For this review, take the finished solid that the model builds, in its own axes (mm). Face numbers are marked on the shaded views. A direction names the side the tool comes from. Round coordinates to 2 decimals unless told otherwise and drop trailing zeros. Write each loop counter-clockwise with the first axis right and the second up, starting at its lowest first coordinate (ties: lowest second). Pieces come first, ordered by that corner, then holes. Notation, with made-up numbers: (62.5, -29.5) -> (95.5, -29.5) arc R9 cw to (95.5, -18.5) -> close; hole circle Ø4 at (-13.5, 29.5). An arc over 180 degrees is marked (long way). Answer as CSV lines item,"result". Start each with the question number.
Item 1: Take a section at A-A on x = 22. Give the boundary of the cut face in (y, z), then the cut area to 3 significant figures.
Item 2: Take a section at B-B on y = 40. Give the boundary of the cut face in (x, z).
Item 3: Machinability: for the marked faces 1, 2, 3, 4 and 5, which of the approach directions +Z, -Z, +X, -X, +Y, -Y give a long, thin tool a straight path to every point of the face, cutting with its end or side? Answer none if there is none.
Item 4: Mouldability with a two-part tool opening along Z and no side actions: class the marked faces 6, 7, 8 and 9 as +Z half, -Z half, draft (parallel to the pull), parting line (faces both ways), or undercut.
Item 5: Take a section at C-C on z = 4. Give the boundary of the cut face in (x, y).
Item 6: Wall thickness on probe 1 along X at (y, z) = (10, 2.5); probe 2 along X at (y, z) = (8.5, 2); probe 3 along Z at (x, y) = (62, 7.5): over which ranges is each line inside the solid? List them lowest first. Write a range as from..to.
Item 7: For pin 1 Ø8 at (y, z) = (3, 22.5) entering from +X; pin 2 Ø11 at (x, z) = (106.5, -26.5) entering from -Y; pin 3 Ø13 at (x, z) = (22, 0) entering from +Y; pin 4 Ø21 at (x, z) = (62, 0) entering from +Y, all flat-tipped, find the tip position at first contact; note any pin that passes through.
Item 8: Take a section at D-D on x = 35. Give the boundary of the cut face in (y, z), then the cut area to 3 significant figures.
```python
from build123d import *

# Parameters (mm, degrees)
F0_W     = 114
F0_H     = 46
F1_DEPTH = 33
F3_R     = 6
F2_R     = 8
F4_DEPTH = 46.001
F5_W     = 14
F5_H     = 10
F6_DEPTH = 66.001
F7_W     = 114
F7_H     = 32
F8_DEPTH = 16


with BuildPart() as f1:
    # F0 (on Top) → F1 (new body, symmetric)
    with BuildSketch(Plane.XY):
        with Locations((57, 23)):
            Rectangle(F0_W, F0_H)
    extrude(amount=F1_DEPTH, both=True)

    # F3
    f3_edges = [f1.edges().sort_by_distance(p)[0] for p in [
        (0, 23, 33),
        (0, 23, -33),
    ]]
    fillet(f3_edges, radius=F3_R)

    # F2 (on face) → F4 (cut, through all)
    with BuildSketch(Plane.XZ):
        Polygon((114, -27), (114, 27), (87, 0), align=None)
        with Locations((22, 0)):
            Circle(F2_R)
        with Locations((62, 0)):
            Circle(F2_R)
    extrude(amount=-F4_DEPTH, mode=Mode.SUBTRACT)

    # F5 (on face) → F6 (cut, through all)
    with BuildSketch(Plane.XY.offset(33)):
        with Locations((107, 5)):
            Rectangle(F5_W, F5_H)
    extrude(amount=-F6_DEPTH, mode=Mode.SUBTRACT)

    # F7 (on face) → F8 (cut)
    with BuildSketch(Plane(origin=(0, 46, 0), x_dir=(-1, 0, 0), z_dir=(0, 1, 0))):
        with Locations((-57, 0)):
            Rectangle(F7_W, F7_H)
    extrude(amount=-F8_DEPTH, mode=Mode.SUBTRACT)


solid = f1.part
```
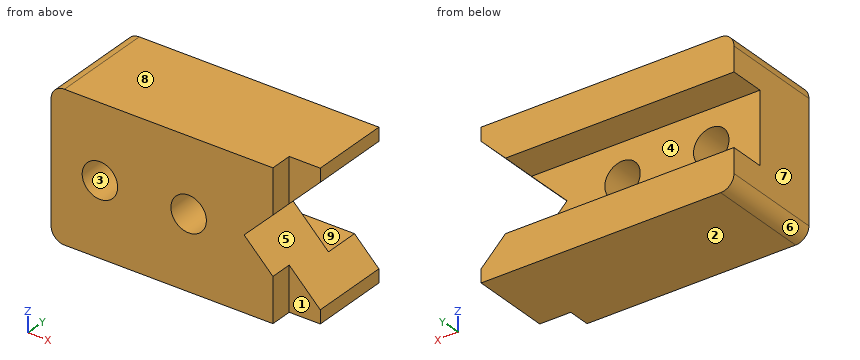
Output values:
1,outline,"(0, -33) -> (46, -33) -> (46, -16) -> (30, -16) -> (30, -8) -> (0, -8) -> close; (0, 8) -> (30, 8) -> (30, 16) -> (46, 16) -> (46, 33) -> (0, 33) -> close"
1,area,"2,040 mm^2"
2,outline,"(0, -27) arc R6 ccw to (6, -33) -> (114, -33) -> (114, -27) -> (103, -16) -> (0, -16) -> close; (0, 16) -> (103, 16) -> (114, 27) -> (114, 33) -> (6, 33) arc R6 ccw to (0, 27) -> close"
3,face 1,"+Z, -Z, +X, -Y"
3,face 2,"-Z, +X, -X, +Y, -Y"
3,face 3,"+Y, -Y"
3,face 4,"+X, -X, +Y"
3,face 5,"+X, +Y, -Y"
4,face 6,"-Z half"
4,face 7,"draft"
4,face 8,"+Z half"
4,face 9,"undercut"
5,outline,"(0, 0) -> (15.07, 0) -> (15.07, 30) -> (0, 30) -> close; (28.93, 0) -> (55.07, 0) -> (55.07, 30) -> (28.93, 30) -> close; (68.93, 0) -> (91, 0) -> (91, 30) -> (68.93, 30) -> close"
6,probe 1,"x = 0..14.4, 29.6..54.4, 69.6..89.5"
6,probe 2,"x = 0..14.25, 29.75..54.25, 69.75..89"
6,probe 3,"z = -33..-8, 8..33"
7,pin 1,"stops at x = 100"
7,pin 2,"stops at y = 10"
7,pin 3,"passes through"
7,pin 4,"stops at y = 30"
8,outline,"(0, -33) -> (46, -33) -> (46, -16) -> (30, -16) -> (30, 16) -> (46, 16) -> (46, 33) -> (0, 33) -> close"
8,area,"2,520 mm^2"
